Check sheet for the modelled part. Datum: model origin and axes. Units: mm. A direction names the side the tool comes from. Give positions to 0.01 mm unless a question says otherwise; leave off trailing zeros. Loops run counter-clockwise (first coordinate to the right, second up) from the corner with the lowest first, then second, coordinate; pieces in that order, holes last. Notation, with made-up numbers: M -10,43 L 23,43 A9 cw 23,55 Z; hole C 24.25,2.5 d9. An arc over 180 degrees is marked long. Use one line per item in the form item = value.
Autodesk Inventor part; units mm, degrees
ref_plane "YZ Plane" through (0, 0, 0) normal (1, 0, 0) x (0, 1, 0)
ref_plane "XZ Plane" through (0, 0, 0) normal (0, 1, 0) x (-1, 0, 0)
ref_plane "XY Plane" through (0, 0, 0) normal (0, 0, 1) x (1, 0, 0)
sketch "Sketch1" plane through (0, 0, 0) normal (0, 1, 0) x (-1, 0, 0)
  line L0 (0, 0) -> (16, 0)
  line L1 (16, 0) -> (16, 40.3)
  line L2 (16, 40.3) -> (0, 40.3)
  line L3 (0, 40.3) -> (0, 0)
  dimension "d0" = 16
  dimension "d1" = 40.3
extrude "Extrusion1" add sketch "Sketch1" along normal blind 4.5
sketch "Sketch2" plane through (0, 4.5, 0) normal (0, 1, 0) x (1, 0, 0)
  line L0 (0, -40.3) -> (0, 0)
  line L1 (0, 0) -> (-6, 0)
  line L2 (0, 0) -> (-16, 0)
  line L3 (-6, 0) -> (-6, -5.825)
  line L4 (-6, -5.825) -> (-6, -13.825)
  line L5 (-6, -13.825) -> (-6, -25.475)
  line L6 (-6, -25.475) -> (-6, -33.475)
  circle A0 centre (-6, -33.475) radius 1.05
  circle A1 centre (-6, -25.475) radius 1.05
  circle A2 centre (-6, -13.825) radius 1.05
  circle A3 centre (-6, -5.825) radius 1.05
  dimension "d4" = 6
  dimension "d5" = 5.825
  dimension "d6" = 8
  dimension "d7" = 11.65
  dimension "d8" = 8
  dimension "d9" = 2.1
  dimension "d10" = 2.1
  dimension "d11" = 2.1
  dimension "d12" = 2.1
extrude "Extrusion2" cut sketch "Sketch2" against normal blind 5
sketch "Sketch3" plane through (0, 4.5, 0) normal (0, 1, 0) x (1, 0, 0)
  circle A0 centre (-6, -5.825) radius 1.05
  circle A1 centre (-6, -5.825) radius 2.5
  circle A2 centre (-6, -13.825) radius 1.05
  circle A3 centre (-6, -13.825) radius 2.5
  circle A4 centre (-6, -25.475) radius 1.05
  circle A5 centre (-6, -25.475) radius 2.5
  circle A6 centre (-6, -33.475) radius 1.05
  circle A7 centre (-6, -33.475) radius 2.5
  point P0 (0, 0)
  dimension "d15" = 5
  dimension "d16" = 5
  dimension "d17" = 5
  dimension "d18" = 5
extrude "Extrusion3" cut sketch "Sketch3" against normal blind 2.2
sketch "Sketch4" plane through (-16, 0, 40.3) normal (0, 0, 1) x (1, 0, 0)
  line L0 (16, 4.5) -> (0, 4.5)
  line L1 (0, 0) -> (16, 0)
  line L2 (16, 0) -> (16, 4.5)
  line L3 (16, 4.5) -> (0, 4.5)
  line L4 (0, 4.5) -> (0, 0)
  point P0 (0, 4.5)
extrude "Extrusion4" cut sketch "Sketch4" against normal blind 1
sketch "Sketch5" plane through (-16, 0, 39.3) normal (0, 0, 1) x (1, 0, 0)
  line L0 (0, 0) -> (0, 4.5)
  line L1 (0, 0) -> (0, 4.5)
  line L2 (0, 4.5) -> (0, 12)
  line L3 (0, 12) -> (4, 12)
  line L4 (4, 12) -> (4, 4.5)
  line L5 (16, 4.5) -> (0, 4.5)
  line L6 (4, 4.5) -> (0, 4.5)
  point P0 (16, 0)
  dimension "d23" = 7.5
  dimension "d24" = 4
extrude "Extrusion5" add sketch "Sketch5" against normal blind 39.3
sketch "Sketch6" plane through (-12, 4.5, 39.3) normal (1, 0, 0) x (0, 0, -1)
  line L0 (39.3, 7.5) -> (39.3, 0)
  line L1 (39.3, 0) -> (39.3, 3)
  line L2 (39.3, 3) -> (29.9, 3)
  line L3 (28.3, 3) -> (12.9, 3)
  line L4 (11.3, 3) -> (3.3, 3)
  arc A0 (1.7, 3) -> (4.3224, 4.2308) centre (3.3, 3) ccw
  arc A1 (9.7, 3) -> (12.9, 3) centre (11.3, 3) ccw
  arc A2 (26.7, 3) -> (29.9, 3) centre (28.3, 3) ccw
  line L5 (3.3, 3) -> (3.3, 6)
  arc A3 (12.5682, 5.0245) -> (10.0318, 5.0245) centre (11.3, 6) ccw
  line L6 (4.9, 6) -> (4.9, 3)
  line L7 (1.7, 6) -> (1.7, 3)
  arc A4 (4.9, 6) -> (1.7, 6) centre (3.3, 6) ccw
  arc A5 (2.4693, 5) -> (3.3, 4.7) centre (3.3, 6) ccw
  line L8 (11.3, 3) -> (11.3, 3.7)
  line L9 (11.3, 4.3) -> (11.3, 6)
  line L10 (28.3, 3) -> (28.3, 3.7)
  line L11 (9.7, 3) -> (9.7, 6)
  line L12 (12.9, 3) -> (12.9, 6)
  line L13 (28.3, 3) -> (28.3, 6)
  arc A6 (29.9, 6) -> (26.7, 6) centre (28.3, 6) ccw
  line L14 (29.9, 3) -> (29.9, 6)
  line L15 (26.7, 3) -> (26.7, 6)
  point P0 (39.3, -4.5)
  dimension "d27" = 3
  dimension "d28" = 11
  dimension "d29" = 17
  dimension "d30" = 8
  dimension "d36" = 3.2
  dimension "d37" = 3.2
  dimension "d38" = 3.2
  dimension "d39" = 3
  dimension "d40" = 3
  dimension "d43" = 3.2
  dimension "d49" = 3
  dimension "d50" = 3.2
extrude "Extrusion6" cut sketch "Sketch6" against normal blind 4.5 contours A0 L7 A4 L6
sketch "Sketch7" plane through (-16, 12, 39.3) normal (0, 1, 0) x (1, 0, 0)
  line L0 (0, 0) -> (0, 39.3)
  line L1 (0, 0) -> (4, 0)
  line L2 (4, 0) -> (4, 39.3)
  line L3 (4, 39.3) -> (0, 39.3)
  line L4 (0, 39.3) -> (0, 0)
  point P0 (16, 39.3)
extrude "Extrusion7" add sketch "Sketch7" along normal blind 1.5
extrude "Extrusion8" cut sketch "Sketch6" along normal mid plane 3 contours A1 L11 A3 L12 | L15 A6 L14 A2
sketch "Sketch8" plane through (0, 0, 0) normal (1, 0, 0) x (0, 0, -1)
  line L0 (0, 0) -> (0, 4.5)
  line L1 (0, 0) -> (0, 4.5)
  line L2 (0, 4.5) -> (0, -3.5)
  line L3 (-39.3, 4.5) -> (0, 4.5)
  line L4 (0, 4.5) -> (-39.3, 4.5)
  line L5 (-39.3, 4.5) -> (-39.3, -3.5)
  line L6 (-39.3, 0) -> (-39.3, 13.5)
  line L7 (-39.3, -3.5) -> (0, -3.5)
  dimension "d53" = 8
extrude "Extrusion9" add sketch "Sketch8" along normal blind 2
sketch "Sketch9" plane through (2, 0, 0) normal (1, 0, 0) x (0, 0, -1)
  line L0 (0, 0) -> (0, 4.5)
  line L1 (0, 4.5) -> (0, -14.5)
  line L2 (0, -14.5) -> (-6, -14.5)
  line L3 (-6, -14.5) -> (-6, 4.5)
  line L4 (-8.325, 4.5) -> (-8.325, 2.3)
  line L5 (0, 4.5) -> (-39.3, 4.5)
  line L6 (-6, 4.5) -> (0, 4.5)
  dimension "d56" = 19
  dimension "d57" = 6
extrude "Extrusion10" add sketch "Sketch9" along normal blind 27
sketch "Sketch10" plane through (-12, 13.5, 0) normal (0, 0, -1) x (-1, 0, 0)
  line L0 (-14, -9) -> (-41, -9)
  line L1 (-41, -9) -> (-36, -9)
  line L2 (-36, -9) -> (-36, -14)
  circle A0 centre (-36, -14) radius 1.9305
  line L3 (-14, -28) -> (-41, -28)
  line L4 (-41, -28) -> (-36, -28)
  line L5 (-36, -28) -> (-36, -23)
  circle A1 centre (-36, -23) radius 1.9305
  point P0 (-12, -13.5)
  dimension "d60" = 5
  dimension "d61" = 5
  dimension "d62" = 3.861
  dimension "d63" = 5
  dimension "d64" = 5
  dimension "d65" = 3.861
extrude "Extrusion11" cut sketch "Sketch10" against normal blind 20
sketch "Sketch11" plane through (-12, 13.5, 0) normal (0, 0, -1) x (-1, 0, 0)
  line L0 (-14, -28) -> (-41, -28)
  line L1 (-14, -28) -> (-19, -28)
  line L2 (-19, -28) -> (-19, -17)
  line L3 (-19, -17) -> (-14, -17)
  line L4 (-14, -17) -> (-14, -28)
  point P0 (-12, -13.5)
  point P1 (-19, -28)
  dimension "d68" = 5
  dimension "d69" = 11
extrude "Extrusion12" cut sketch "Sketch11" against normal blind 25
sketch "Sketch12" plane through (-13.5, 4.5, 39.3) normal (1, 0, 0) x (0, 0, -1)
  arc A0 (12.9, 6) -> (9.7, 6) centre (11.3, 6) ccw
  circle A1 centre (11.3, 6) radius 1.6
  arc A2 (9.7, 3) -> (12.9, 3) centre (11.3, 3) ccw
  circle A3 centre (11.3, 3) radius 1.6
  line L0 (9.7, 3) -> (9.7, 6)
  line L1 (9.7, 6) -> (9.7, 3)
  line L2 (12.9, 6) -> (12.9, 3)
  line L3 (12.9, 6) -> (12.9, 3)
  arc A4 (26.7, 3) -> (29.9, 3) centre (28.3, 3) ccw
  line L4 (11.3, 3) -> (28.3, 3)
  line L5 (28.3, 3) -> (19.8, 3)
  line L6 (19.8, 3) -> (19.8, 4.3)
  arc A5 (29.9, 6) -> (26.7, 6) centre (28.3, 6) ccw
  circle A6 centre (28.3, 6) radius 1.6
  circle A7 centre (28.3, 3) radius 1.6
  line L7 (29.9, 3) -> (29.9, 6)
  line L8 (29.9, 6) -> (29.9, 3)
  line L9 (26.7, 6) -> (26.7, 3)
  line L10 (26.7, 6) -> (26.7, 3)
  point P0 (39.3, -4.5)
extrude "Extrusion13" cut sketch "Sketch12" against normal blind 3
sketch "Sketch13" plane through (-12, 4.5, 39.3) normal (1, 0, 0) x (0, 0, -1)
  arc A0 (4.9, 6) -> (3.8568, 7.5) centre (3.3, 6) ccw
  circle A1 centre (3.3, 6) radius 1.6
  point P0 (39.3, -4.5)
  point P1 (4.9, 6)
  dimension "d74" = 3.2
extrude "Extrusion14" cut sketch "Sketch13" along normal mid plane 8
properties part number "Non_compliant_plate"
1) Scan lines: line 1 (Z direction, x = -6, y = 0.9) (3 decimals); line 2 (Y direction, x = 24, z = 4); line 3 (Z direction, x = -14, y = 7.5). Record each from-to range of solid material in increasing order.
Evaluation:
line_1 = 0 to 4.775, 6.875 to 12.775, 14.875 to 24.425, 26.525 to 32.425, 34.525 to 39.3
line_2 = -14.5 to -11.43, -7.57 to -2.43, 1.43 to 4.5
line_3 = 0 to 9.4, 12.6 to 26.4, 29.6 to 34.4, 37.6 to 39.3
2) Section check A-A (y = -9.5). Record the cut outline in (x, z), then the cut area to 3 significant figures.
Evaluation:
outline = M 7,0 L 22.07,0 L 22.07,6 L 7,6 Z; M 25.93,0 L 29,0 L 29,6 L 25.93,6 Z
area = 109 mm^2
3) Section check B-B (z = 17). Record the cut outline in (x, y).
Evaluation:
outline = M -16,0 L 0,0 L 0,-3.5 L 2,-3.5 L 2,4.5 L -12,4.5 L -12,13.5 L -16,13.5 Z
4) Depth check by flat-ended pin: pin 1 Ø7.5 at (x, z) = (3.5, 14) entering from -Y; pin 2 Ø2 at (x, y) = (6.5, -7) entering from +Z; pin 3 Ø2 at (y, z) = (-2, 14.5) entering from +X. Enter the tip coordinate at first touch or a pass-through.
Evaluation:
pin_1 = -3.5
pin_2 = 6
pin_3 = 2
5) Set-up check for faces 1 (the face through (2, 1, 23)), 2 (the face through (0, -2, 20)), 3 (the face through (-5, 2.3, 7)), 4 (the face through (1, 4.5, 15)), 5 (the face through (-14, 12.1, 11)): record each of +Z, -Z, +X, -X, +Y, -Y from which the full face is reachable in a straight line by a thin tool's end or side.
Evaluation:
face_1 = +Z, +X, +Y, -Y
face_2 = +Z, -Z, -X, -Y
face_3 = +Y
face_4 = +Z, -Z, +X, +Y
face_5 = +X, -X
6) Section check C-C (z = 10.5). Record the cut outline in (x, y), then the cut area to 3 significant figures.
Evaluation:
outline = M -16,0 L 0,0 L 0,-3.5 L 2,-3.5 L 2,4.5 L -12,4.5 L -12,5.98 L -16,5.98 Z; M -16,12.02 L -12,12.02 L -12,13.5 L -16,13.5 Z
area = 99.8 mm^2
7) Section check D-D (x = -6). State how many separate pieces and enclosed holes the cut face has, then the cut area to 3 significant figures.
Evaluation:
separate_pieces = 5
enclosed_holes = 0
area = 114 mm^2
8) Release check for a two-part mould opening along Z. For faces 6 (the face through (11, -3, 0)), 7 (the face through (-12.8, 12.1, 28)), 8 (the face through (7, -9, 3)) record: pulls with the +Z half, pulls with the -Z half, needs draft (parallel to the pull), parting line crosses it, or undercut.
Evaluation:
face_6 = pulls with the -Z half
face_7 = undercut
face_8 = needs draft
